from build123d import *

# Parameters (mm, degrees)
SKETCH2_R               = 44.45
BOSS_EXTRUDE1_DEPTH     = 4.7625
F_6_CLEARANCE_HOLE1_D   = 3.7973
CIRPATTERN1_COUNT       = 4
CUT_EXTRUDE1_DEPTH      = 64.041941644
CUT_EXTRUDE1_DEPTH_BACK = 64.041941644


with BuildPart() as part:
    # Sketch2 → Boss-Extrude1 (new body)
    with BuildSketch(Plane.XY):
        with Locations(Location((0, 0, 0), (0, 0, 180))):
            Circle(SKETCH2_R)
    extrude(amount=BOSS_EXTRUDE1_DEPTH)

    # #6 Clearance Hole1 (through all)
    with Locations(Plane.XY.offset(4.7625)):
        with Locations((0, 42.06875)):
            f_6_clearance_hole1 = Hole(F_6_CLEARANCE_HOLE1_D / 2)

    # CirPattern1: #6 Clearance Hole1 ×4 about axis
    cirpattern1_axis = Axis((0, 0, 0), (0, 0, 1))
    for i in range(1, CIRPATTERN1_COUNT):
        add(f_6_clearance_hole1.rotate(cirpattern1_axis, i * 360 / CIRPATTERN1_COUNT), mode=Mode.SUBTRACT)

    # Sketch5 → Cut-Extrude1 (cut, two sides: drawn at the far end of the back side and taken through both)
    with BuildSketch(Plane.XY.offset(4.7625).offset(-CUT_EXTRUDE1_DEPTH_BACK)):
        with BuildLine():
            Line((16.539365803, -41.367349975), (13.001856878, -34.261722849))
            ThreePointArc((13.001856878, -34.261722849), (13.715480519, -32.133095639), (15.844107729, -32.846719279))
            Line((15.844107729, -32.846719279), (19.381616653, -39.952346405))
            ThreePointArc((19.381616653, -39.952346405), (18.667993013, -42.080973615), (16.539365803, -41.367349975))
        make_face()
    extrude(amount=CUT_EXTRUDE1_DEPTH + CUT_EXTRUDE1_DEPTH_BACK, mode=Mode.SUBTRACT)


solid = part.part
Source: CAD feature listing. Evaluate the final solid. Frame: model axes, mm. A direction names the side the tool comes from. Coordinates: 2 decimals unless noted, no trailing zeros. Order: outer loops, then holes, each group sorted by start corner. A loop starts at its lowest first (then second) coordinate and runs counter-clockwise, first axis right, second up.
Item 1: Set-up query: faces 1 (the face through (17.59, -36.35, 2.35)), 2 (the face through (1, -1, 0)). Return all of +Z, -Z, +X, -X, +Y, -Y with unobstructed straight access to the full face (end or side cutting, diameter ignored); none if empty.
Output values:
face 1: +Z, -Z
face 2: -Z, +X, -X, +Y, -Y
Item 2: Material intervals for line 1 (Y direction, x = 0, z = 3); line 2 (Y direction, x = 13.5, z = 3.6); line 3 (X direction, y = 20, z = 3.25), sorted ascending.
Output values:
line 1: y = -44.45 to -43.97, -40.17 to 40.17, 43.97 to 44.45
line 2: y = -42.35 to -35.26, -32.26 to 42.35
line 3: x = -39.7 to 39.7
Item 3: Cut plane C-C (y = 21.5). Return loops of the section in (x, z), plus the area to 3 significant figures.
Output values:
outline: (-38.9, 0) - (38.9, 0) - (38.9, 4.76) - (-38.9, 4.76) - close
area: 371 mm2
Item 4: Cut plane A-A (x = 0). Return loops of the section in (y, z), plus the area to 3 significant figures.
Output values:
outline: (-44.45, 0) - (-43.97, 0) - (-43.97, 4.76) - (-44.45, 4.76) - close; (-40.17, 0) - (40.17, 0) - (40.17, 4.76) - (-40.17, 4.76) - close; (43.97, 0) - (44.45, 0) - (44.45, 4.76) - (43.97, 4.76) - close
area: 387 mm2
Item 5: First-contact query: P1, Ø1.5, axis at x = -32, z = 1.5, coming from the +Y side; P2, Ø3, axis at x = 0, y = 42.07, coming from the +Z side. Flat tips, straight axial feed; report the tip coordinate or a pass-through.
Output values:
P1: stops at y = 31.61
P2: passes through
Item 6: Cut plane B-B (z = 1.9). Count the separate pieces of the cut face and the enclosed holes in it, plus the area to 3 significant figures.
Output values:
separate pieces: 1
enclosed holes: 4
area: 6,130 mm2
Item 7: Cut plane D-D (x = -20.5). Return loops of the section in (y, z), plus the area to 3 significant figures.
Output values:
outline: (-39.44, 0) - (39.44, 0) - (39.44, 4.76) - (-39.44, 4.76) - close
area: 376 mm2
Item 8: Pull-direction query (Y, two-part tool) for faces 3 (the face through (14.772, -37.818, 2.348)), 4 (the face through (-40.384, -0.876, 2.348)), 5 (the face through (1, -1, 4.762)); classes: pulls with the +Y half, pulls with the -Y half, needs draft (parallel to the pull), parting line crosses it, or undercut.
Output values:
face 3: undercut
face 4: undercut
face 5: needs draft
